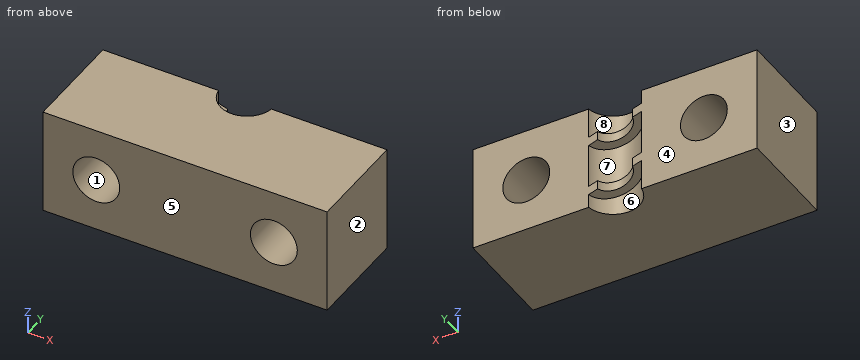
```python
from build123d import *

# Parameters (mm, degrees)
SKETCH_1_W               = 16
SKETCH_1_H               = 12
SKETCH_1_R               = 1.5
EXTRUDE_1_DEPTH          = 3
EXTRUDE_2_DEPTH          = 6
CUT_EXTRUDE_2_DEPTH      = 11.440306509
CUT_EXTRUDE_2_DEPTH_BACK = 11.440306509
SKETCH_8_R               = 1.32
CUT_EXTRUDE_3_DEPTH      = 11.440306509


with BuildPart() as part:
    # 草图1 → 凸台-拉伸1 (new, symmetric)
    with BuildSketch(Plane.XY):
        Rectangle(SKETCH_1_W, SKETCH_1_H)
        Circle(SKETCH_1_R, mode=Mode.SUBTRACT)
    extrude(amount=EXTRUDE_1_DEPTH, both=True)

    # 草图6 → 凸台-拉伸2 (add)
    with BuildSketch(Plane(origin=(0, 0, 0), x_dir=(1, 0, 0), z_dir=(0, 1, 0))):
        Polygon((-1.5, -1.727557465), (-1.5, -2.227557465), (1.5, -1.272442535), (1.5, -0.772442535), align=None)
        Polygon((-1.5, 1.272442535), (-1.5, 0.772442535), (1.5, 1.727557465), (1.5, 2.227557465), align=None)
    extrude(amount=-EXTRUDE_2_DEPTH)

    # 草图7 → 切除-拉伸2 (cut, two sides: drawn at the far end of the back side and taken through both)
    with BuildSketch(Plane.XY.offset(-CUT_EXTRUDE_2_DEPTH_BACK)):
        with BuildLine():
            Line((-8, -0.203898058), (-0.978992126, -0.203898058))
            ThreePointArc((-0.978992126, -0.203898058), (-0.102488717, 0.994734167), (1, 0))
            ThreePointArc((1, 0), (0.994734167, -0.102488717), (0.978992126, -0.203898058))
            Line((0.978992126, -0.203898058), (8, -0.203898058))
            Line((8, -0.203898058), (8, 6))
            Line((8, 6), (-8, 6))
            Line((-8, 6), (-8, -0.203898058))
        make_face()
        with BuildLine():
            Line((0.978992126, -0.203898058), (0, 0))
            Line((0, 0), (-0.978992126, -0.203898058))
            ThreePointArc((-0.978992126, -0.203898058), (0, -1), (0.978992126, -0.203898058))
        make_face()
        with BuildLine():
            Line((-0.978992126, -0.203898058), (0, 0))
            Line((0, 0), (0.978992126, -0.203898058))
            ThreePointArc((0.978992126, -0.203898058), (0.994734167, -0.102488717), (1, 0))
            ThreePointArc((1, 0), (-0.102488717, 0.994734167), (-0.978992126, -0.203898058))
        make_face()
    extrude(amount=CUT_EXTRUDE_2_DEPTH + CUT_EXTRUDE_2_DEPTH_BACK, mode=Mode.SUBTRACT)

    # 草图8 → 切除-拉伸3 (cut, through all)
    with BuildSketch(Plane(origin=(0, 0, 0), x_dir=(1, 0, 0), z_dir=(0, 1, 0))):
        with Locations(Location((-5, 0, 0), (0, 0, 270))):
            Circle(SKETCH_8_R)
        with Locations(Location((5, 0, 0), (0, 0, 270))):
            Circle(SKETCH_8_R)
    extrude(amount=-CUT_EXTRUDE_3_DEPTH, mode=Mode.SUBTRACT)


solid = part.part
```
For this review, take the finished solid that the model builds, in its own axes (mm). Face numbers are marked on the shaded views. A direction names the side the tool comes from. Coordinates: 2 decimals unless noted, no trailing zeros. Order: outer loops, then holes, each group sorted by start corner. A loop starts at its lowest first (then second) coordinate and runs counter-clockwise, first axis right, second up. Notation, with made-up numbers: (64.25, 16.25) -> (99.25, 16.25) arc R19 ccw to (99.25, 29.25) -> close; hole circle Ø4 at (33.5, 4). An arc over 180 degrees is marked (long way). Answer as CSV lines item,"result".
Q1. We need section B-B (x = -5). State the section outline as (y, z) points.
Model answer:
outline,"(-6, -3) -> (-0.2, -3) -> (-0.2, -1.32) -> (-6, -1.32) -> close; (-6, 1.32) -> (-0.2, 1.32) -> (-0.2, 3) -> (-6, 3) -> close"
Q2. Draft analysis for pull direction X (two halves, no side actions). For the marked faces 1, 2 and 3, state which applies: released by +X, released by -X, zero draft, split by the parting line, or undercut.
Model answer:
face 1,"undercut"
face 2,"released by +X"
face 3,"released by -X"
Q3. For the marked faces 4, 5, 6, 7 and 8, list the 3-axis set-ups (+Z, -Z, +X, -X, +Y, -Y) from which the entire face can be reached by the end or side of a thin tool; tool diameter is ignored.
Model answer:
face 4,"+Z, -Z, +X, -X, +Y"
face 5,"+Z, -Z, +X, -X, -Y"
face 6,"-Z, +Y"
face 7,"+Y"
face 8,"+Z, +Y"
Q4. Wall thickness on line 1 along X through (y, z) = (-2.4, 0); line 2 along X through (y, z) = (-2.45, 1.1); line 3 along X through (y, z) = (-0.7, -0.4): over which ranges is each line inside the solid? List them lowest first. Write a range as [from, to].
Model answer:
line 1,"x = [-8, -6.32], [-3.68, 3.68], [6.32, 8]"
line 2,"x = [-8, -5.73], [-4.27, 4.27], [5.73, 8]"
line 3,"x = [-8, -6.26], [-3.74, -1.33], [1.33, 3.74], [6.26, 8]"
Q5. We need section D-D (x = 4). State the section outline as (y, z) points.
Model answer:
outline,"(-6, -3) -> (-0.2, -3) -> (-0.2, -0.86) -> (-6, -0.86) -> close; (-6, 0.86) -> (-0.2, 0.86) -> (-0.2, 3) -> (-6, 3) -> close"
Q6. We need section A-A (z = 0). State the section outline as (x, y) points, plus the area to 3 significant figures.
Model answer:
outline,"(-8, -6) -> (-6.32, -6) -> (-6.32, -0.2) -> (-8, -0.2) -> close; (-3.68, -6) -> (3.68, -6) -> (3.68, -0.2) -> (1.49, -0.2) arc R1.5 cw to (-1.49, -0.2) -> (-3.68, -0.2) -> close; (6.32, -6) -> (8, -6) -> (8, -0.2) -> (6.32, -0.2) -> close"
area,"59.2 mm2"
Q7. We need section C-C (y = -2.65). State the section outline as (x, z) points, plus the area to 3 significant figures.
Model answer:
outline,"(-8, -3) -> (8, -3) -> (8, 3) -> (-8, 3) -> close; hole circle Ø2.64 at (-5, 0); hole circle Ø2.64 at (5, 0)"
area,"85.1 mm2"
